The listing builds one solid part. Answer for the finished solid, in the listing's coordinates (mm). Face numbers are marked on the shaded views. Coordinates: 2 decimals unless noted, no trailing zeros. Loops run counter-clockwise (first coordinate to the right, second up) from the corner with the lowest first, then second, coordinate; pieces in that order, holes last. Notation, with made-up numbers: M 8,0 L 35,0 A19 ccw 35,30 Z; hole C 27.5,-24 d5. An arc over 180 degrees is marked long. Answer as a JSON object with one key per item and string values. Group by question number.
1. A cutting plane is placed at B-B on y = 12.7. Give the vertices of the cut face in (x, z), and give its area (3 significant figures).
2. Determine the mould class of the marked faces 1, 2, 3 and 4 for opening direction Z: released by +Z, released by -Z, zero draft, split by the parting line, or undercut.
3. A cutting plane is placed at C-C on x = 14.25. Give the vertices of the cut face in (y, z).
4. Given pin 1 (1.7 mm diameter, centred on x = 17.5, y = 14.5, fed in from +Z); pin 2 (3.5 mm diameter, centred on y = 12.7, z = -6.731, fed in from -X); pin 3 (2 mm diameter, centred on y = 11.5, z = -6.5, fed in from +X), each flat-ended and moving along its own axis, determine where each tip first touches the part or whether it passes through.
5. Straight lines are drawn through the part: L1, parallel to Y at x = 16.5, z = -4.5; L2, parallel to Y at x = 13, z = -8; L3, parallel to Z at x = 10, y = 46. For each, find the intervals that lie inside material, in ascending order.
6. A cutting plane is placed at A-A on x = 2.75. Give the vertices of the cut face in (y, z).
7. A cutting plane is placed at D-D on y = 28.5. Give the vertices of the cut face in (x, z), and give its area (3 significant figures).
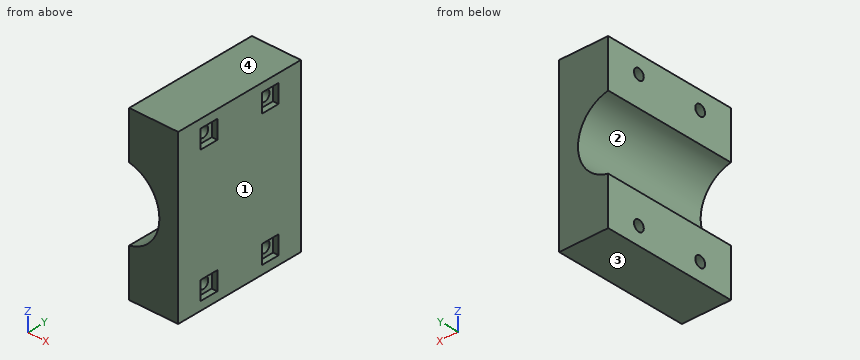
from build123d import *

# Parameters (mm, degrees)
SKETCH1_W           = 18.542
SKETCH1_H           = 63.5
BOSS_EXTRUDE1_DEPTH = 50.8
CUT_EXTRUDE1_DEPTH  = 50.8
SKETCH4_R           = 2.032
CUT_EXTRUDE3_DEPTH  = 18.542
CUT_EXTRUDE4_START  = -2.0955
SKETCH6_W           = 6.985
SKETCH6_H           = 6.985
CUT_EXTRUDE4_DEPTH  = 2.0955


with BuildPart() as part:
    # Sketch1 → Boss-Extrude1 (new body)
    with BuildSketch(Plane(origin=(0, 0, 0), x_dir=(1, 0, 0), z_dir=(0, 1, 0))):
        with Locations((9.271, 31.75)):
            Rectangle(SKETCH1_W, SKETCH1_H)
    extrude(amount=BOSS_EXTRUDE1_DEPTH)

    # Sketch2 → Cut-Extrude1 (cut)
    with BuildSketch(Plane(origin=(0, 50.8, 0), x_dir=(1, 0, 0), z_dir=(0, 1, 0))):
        with BuildLine():
            Line((-2.54, 45.72), (-2.54, 17.78))
            ThreePointArc((-2.54, 17.78), (11.43, 31.75), (-2.54, 45.72))
        make_face()
    extrude(amount=-CUT_EXTRUDE1_DEPTH, mode=Mode.SUBTRACT)

    # Sketch4 → Cut-Extrude3 (cut)
    with BuildSketch(Plane(origin=(18.542, 0, 0), x_dir=(0, 0, -1), z_dir=(1, 0, 0))):
        with Locations((56.769, 38.1)):
            Circle(SKETCH4_R)
        with Locations((56.769, 12.7)):
            Circle(SKETCH4_R)
        with Locations((6.731, 38.1)):
            Circle(SKETCH4_R)
        with Locations((6.731, 12.7)):
            Circle(SKETCH4_R)
    extrude(amount=-CUT_EXTRUDE3_DEPTH, mode=Mode.SUBTRACT)

    # Sketch6 → Cut-Extrude4 (cut)
    with BuildSketch(Plane(origin=(18.542, 0, 0), x_dir=(0, 0, -1), z_dir=(1, 0, 0)).offset(CUT_EXTRUDE4_START)):
        with Locations((56.769, 38.1)):
            Rectangle(SKETCH6_W, SKETCH6_H)
        with Locations((56.769, 12.7)):
            Rectangle(SKETCH6_W, SKETCH6_H)
        with Locations((6.731, 38.1)):
            Rectangle(SKETCH6_W, SKETCH6_H)
        with Locations((6.731, 12.7)):
            Rectangle(SKETCH6_W, SKETCH6_H)
    extrude(amount=CUT_EXTRUDE4_DEPTH, mode=Mode.SUBTRACT)


solid = part.part
From the geometry:
{
 "1": {"outline": "M 0,-63.5 L 18.54,-63.5 L 18.54,-60.26 L 16.45,-60.26 L 16.45,-58.8 L 0,-58.8 Z; M 0,-54.74 L 16.45,-54.74 L 16.45,-53.28 L 18.54,-53.28 L 18.54,-10.22 L 16.45,-10.22 L 16.45,-8.76 L 0,-8.76 L 0,-18.01 A13.97 cw 0,-45.49 Z; M 0,-4.7 L 16.45,-4.7 L 16.45,-3.24 L 18.54,-3.24 L 18.54,0 L 0,0 Z", "area": "778 mm²"},
 "2": {"face 1": "zero draft", "face 2": "undercut", "face 3": "released by -Z", "face 4": "released by +Z"},
 "3": {"outline": "M 0,-63.5 L 50.8,-63.5 L 50.8,0 L 0,0 Z; hole C 12.7,-56.77 d4.06; hole C 12.7,-6.73 d4.06; hole C 38.1,-56.77 d4.06; hole C 38.1,-6.73 d4.06"},
 "4": {"pin 1": "stops at z = 0", "pin 2": "passes through", "pin 3": "stops at x = 16.45"},
 "5": {"L1": "y = 0 to 9.21, 16.19 to 34.61, 41.59 to 50.8", "L2": "y = 0 to 11.11, 14.29 to 36.51, 39.69 to 50.8", "L3": "z = -63.5 to -37.91, -25.59 to 0"},
 "6": {"outline": "M 0,-63.5 L 50.8,-63.5 L 50.8,-44.68 L 0,-44.68 Z; M 0,-18.82 L 50.8,-18.82 L 50.8,0 L 0,0 Z; hole C 12.7,-56.77 d4.06; hole C 12.7,-6.73 d4.06; hole C 38.1,-56.77 d4.06; hole C 38.1,-6.73 d4.06"},
 "7": {"outline": "M 0,-63.5 L 18.54,-63.5 L 18.54,0 L 0,0 L 0,-18.01 A13.97 cw 0,-45.49 Z", "area": "941 mm²"}
}
